Autodesk Inventor part; units mm, degrees
ref_plane "YZ Plane" through (0, 0, 0) normal (1, 0, 0) x (0, 1, 0)
ref_plane "XZ Plane" through (0, 0, 0) normal (0, 1, 0) x (-1, 0, 0)
ref_plane "XY Plane" through (0, 0, 0) normal (0, 0, 1) x (1, 0, 0)
sketch "Sketch1" plane through (0, 0, 0) normal (1, 0, 0) x (0, 1, 0)
  line L0 (0, 0) -> (10, 0)
  line L1 (0, 0) -> (0, -35)
  line L2 (0, -35) -> (10, 0)
  dimension "d0" = 10
  dimension "d1" = 35
extrude "Extrusion1" add sketch "Sketch1" along normal blind 20
sketch "Sketch2" plane through (0, 0, -35) normal (0, -1, 0) x (1, 0, 0)
  line L0 (0, 35) -> (20, 35)
  circle A0 centre (18, 33) radius 1.2
  line L1 (0, 35) -> (0, 0)
  circle A1 centre (2, 33) radius 1.2
  line L2 (20, 35) -> (20, 0)
  circle A2 centre (18, 2) radius 1.2
  circle A3 centre (2, 2) radius 1.2
  dimension "d6" = 2.4
  dimension "d8" = 2.4
  dimension "d12" = 2.4
  dimension "d13" = 2.4
extrude "Extrusion2" cut sketch "Sketch2" against normal through all
sketch "Sketch3" plane through (0, 10, 0) normal (0, 0.9615239, -0.2747211) x (1, 0, 0)
  line L0 (0, 2.7472) -> (0, 36.4005)
  line L1 (0, 36.4005) -> (0, 32.4005)
  line L2 (20, 2.7472) -> (20, 36.4005)
  line L3 (0, 32.4005) -> (20, 32.4005)
  line L4 (20, 32.4005) -> (20, 31.4005)
  line L5 (20, 31.4005) -> (0, 31.4005)
  line L6 (0, 31.4005) -> (0, 32.4005)
  dimension "d16" = 4
  dimension "d17" = 1
extrude "Extrusion3" add sketch "Sketch3" along normal blind 3
properties part number "1_mm_slant"
Could you check a few things on this model? Use its own coordinates, in mm. A direction names the side the tool comes from. Give positions to 0.01 mm unless a question says otherwise; leave off trailing zeros. Write each loop counter-clockwise with the first axis right and the second up, starting at its lowest first coordinate (ties: lowest second). Pieces come first, ordered by that corner, then holes. Notation, with made-up numbers: (-30, 47.5) -> (6, 47.5) arc R28 cw to (6, 72.5) -> close; hole circle Ø4 at (-35.75, 9.5). An arc over 180 degrees is marked (long way). Answer as a JSON object with one key per item and string values.
Q1. Please list where these lines run through material, in increasing order: L1, parallel to X at y = 5.25, z = -2; L2, parallel to Z at x = 18, y = 0.4; L3, parallel to Y at x = 8.25, z = -19.
Taken from the geometry:
{"L1": "x = 0 to 0.8, 3.2 to 16.8, 19.2 to 20", "L2": "z = -31.8 to -3.2, -0.8 to 0", "L3": "y = 0 to 4.57"}
Q2. Suppose I cut it at A-A on z = -33. Write out the boundary of the cut face in (x, y).
Taken from the geometry:
{"outline": "(0, 0) -> (0.8, 0) -> (0.8, 0.57) -> (0, 0.57) -> close; (3.2, 0) -> (16.8, 0) -> (16.8, 0.57) -> (3.2, 0.57) -> close; (19.2, 0) -> (20, 0) -> (20, 0.57) -> (19.2, 0.57) -> close"}
Q3. Which directions (+Z, -Z, +X, -X, +Y, -Y) give clear straight access to the entire face, cutting with the end or side of a thin tool? Please do faces 1 (the flat face through (9.86, 2.52, -31.56)), 2 (the flat face through (10, 0, -17)), 3 (the flat face through (10.1, 2.8, -30.6)), 4 (the flat face through (10, 5, 0)), 5 (the cylindrical face through (17.84, 0.35, -31.81)).
Taken from the geometry:
{"face 1": "-Z, +X, -X", "face 2": "+Z, -Z, +X, -X, -Y", "face 3": "+X, -X, +Y", "face 4": "+Z, +X, -X, +Y, -Y", "face 5": "-Y"}
Q4. Will these pins go through, and if not, where does the flat tip stop? pin 1 Ø2 at (x, z) = (2, -2) entering from -Y; pin 2 Ø4 at (x, z) = (2, -33) entering from +Y; pin 3 Ø4 at (x, y) = (12, 5) entering from -Z.
Taken from the geometry:
{"pin 1": "passes through", "pin 2": "stops at y = 4.26", "pin 3": "stops at z = -31.98"}
Q5. We'd pull the mould along X, two halves only. Please class faces 6 (the flat face through (9.86, 4.12, -31.5)), 7 (the flat face through (20, 4, -13)), 8 (the cylindrical face through (1.84, 0.35, -31.81)), 9 (the cylindrical face through (17.84, 4.82, -0.81)): released by +X, released by -X, zero draft, split by the parting line, or undercut.
Taken from the geometry:
{"face 6": "zero draft", "face 7": "released by +X", "face 8": "undercut", "face 9": "undercut"}
Q6. Suppose I cut it at D-D on x = 6.5. Write out the boundary of the cut face in (y, z).
Taken from the geometry:
{"outline": "(0, -35) -> (1.1, -31.15) -> (3.98, -31.98) -> (4.26, -31.02) -> (1.37, -30.19) -> (10, 0) -> (0, 0) -> close"}
Q7. Suppose I cut it at B-B on x = 18.5. Write out the boundary of the cut face in (y, z), then the cut area to 3 significant figures.
Taken from the geometry:
{"outline": "(0, -35) -> (0.26, -34.09) -> (0, -34.09) -> close; (0, -31.91) -> (0.88, -31.91) -> (1.1, -31.15) -> (3.98, -31.98) -> (4.26, -31.02) -> (1.37, -30.19) -> (9.12, -3.09) -> (0, -3.09) -> close; (0, -0.91) -> (9.74, -0.91) -> (10, 0) -> (0, 0) -> close", "area": "156 mm²"}
Q8. Suppose I cut it at C-C on y = 5.75. Write out the boundary of the cut face in (x, z) (3 decimals).
Taken from the geometry:
{"outline": "(0, -14.875) -> (20, -14.875) -> (20, 0) -> (0, 0) -> close; hole circle Ø2.4 at (2, -2); hole circle Ø2.4 at (18, -2)"}
